Answer from the drawing. Dimensions are ordinates in mm from the lowest x, y and z of the part. A direction names the side the tool comes from. Round coordinates to 2 decimals unless told otherwise and drop trailing zeros. Write each loop counter-clockwise with the first axis right and the second up, starting at its lowest first coordinate (ties: lowest second). Pieces come first, ordered by that corner, then holes. Notation, with made-up numbers: (15.25, 53) -> (40.25, 53) arc R22 ccw to (40.25, 68) -> close; hole circle Ø11 at (39, 69). An arc over 180 degrees is marked (long way). Answer as a JSON object with one key per item and string values. Group by question number.
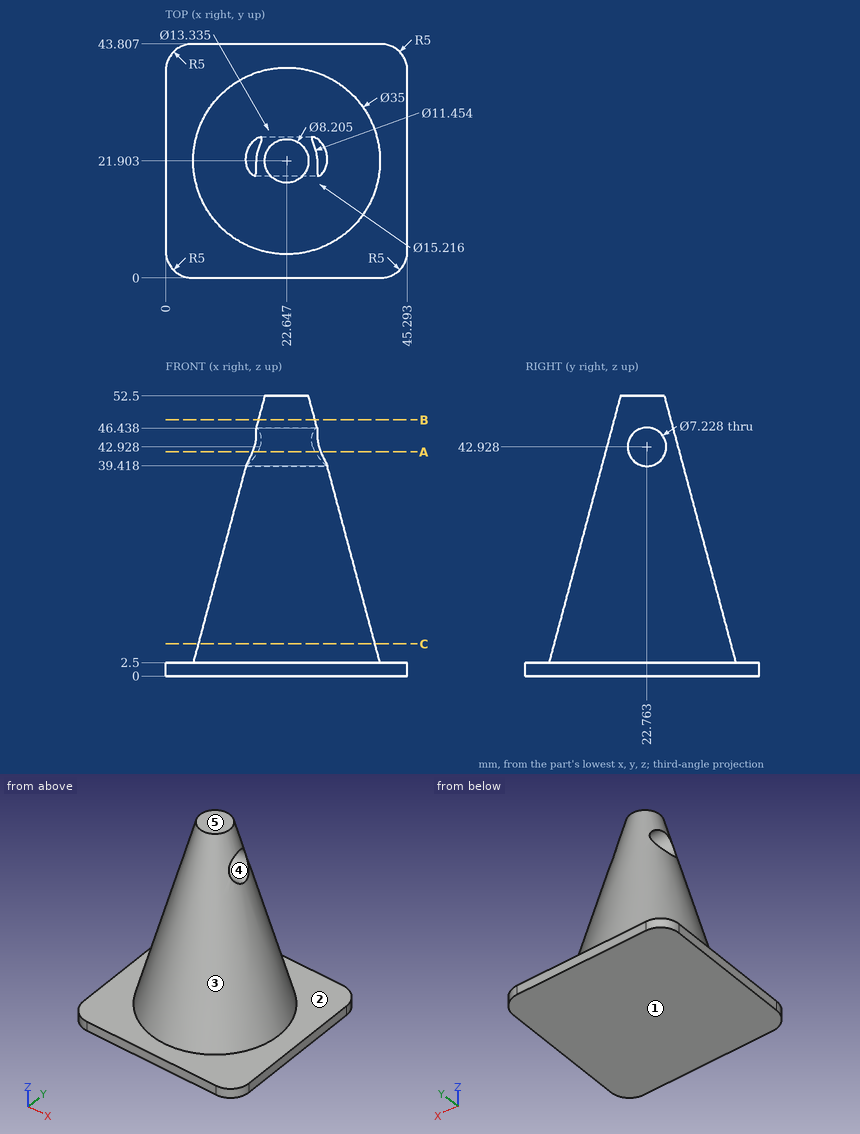
1) A tool of negligible diameter and unlimited length cuts with its end or side. For the marked faces 1 and 2, from which of +Z, -Z, +X, -X, +Y, -Y can it reach the whole face along a straight path? Write none if from no direction.
2) For a pull along Y with two mould halves and no side action, classify the marked faces 3, 4 and 5 as released by +Y, released by -Y, zero draft, split by the parting line, or undercut.
3) A cutting plane is placed at B-B on z = 48. Determine the outline of the cut face in (x, y) (1 decimal).
4) Each of these flat-tipped pins is pushed along its axis until it touches: P1, Ø11.5, axis at y = 22.76, z = 42.93, coming from the +X side; P2, Ø3, axis at x = 17, z = 46, coming from the -Y side. Where does it stop, or does it pass through?
5) Straight lines are drawn through the part: L1, parallel to Z at x = 11, y = 5; L2, parallel to Z at x = 16, y = 22 (1 decimal); L3, parallel to Y at x = 25, z = 38.5 (1 decimal). For each, find the intervals that lie inside material, in ascending order.
6) A cutting plane is placed at A-A on z = 42. Determine the outline of the cut face in (x, y) (1 decimal).
7) A cutting plane is placed at C-C on z = 6. Determine the outline of the cut face in (x, y) (1 decimal).
Established:
{
 "1": {"face 1": "-Z, +X, -X, +Y, -Y", "face 2": "+Z"},
 "2": {"face 3": "split by the parting line", "face 4": "undercut", "face 5": "zero draft"},
 "3": {"outline": "circle Ø10.6 at (22.6, 21.9)"},
 "4": {"P1": "stops at x = 30.84", "P2": "stops at y = 17.68"},
 "5": {"L1": "z = 0 to 2.5", "L2": "z = 0 to 39.4", "L3": "y = 14.4 to 29.4"},
 "6": {"outline": "(16.3, 19.3) arc R6.9 ccw to (29, 19.3) -> close; (17.3, 26.3) -> (28, 26.3) arc R6.9 ccw to start"},
 "7": {"outline": "circle Ø33.1 at (22.6, 21.9)"}
}
